Verification items for the finished model (mm, model axes). Face numbers are marked on the shaded views. A direction names the side the tool comes from. Coordinates: 2 decimals unless noted, no trailing zeros. Write each loop counter-clockwise with the first axis right and the second up, starting at its lowest first coordinate (ties: lowest second). Pieces come first, ordered by that corner, then holes. Notation, with made-up numbers: M 47.25,39.25 L 66.25,39.25 A24 ccw 66.25,66.25 Z; hole C 58.25,-12.75 d9. An arc over 180 degrees is marked long. Answer in a Markdown table with one row per item.
from build123d import *

# Parameters (mm, degrees)
EXTRUDE_1_DEPTH = 27.6


with BuildPart() as part:
    # 草图1 → 凸台-拉伸1 (new body)
    with BuildSketch(Plane.XY):
        with BuildLine():
            Line((13.366208682, 26.400087715), (20.217636418, 24.133453872))
            ThreePointArc((20.217636418, 24.133453872), (23.645978989, 21.408723367), (24.49520491, 17.112619964))
            Line((24.49520491, 17.112619964), (20.150640538, -10.351388685))
            ThreePointArc((20.150640538, -10.351388685), (17.326686466, -15.395594315), (11.903196789, -17.396715696))
            Line((11.903196789, -17.396715696), (-13.656803211, -17.396715696))
            ThreePointArc((-13.656803211, -17.396715696), (-19.080292887, -15.395594315), (-21.90424696, -10.351388685))
            Line((-21.90424696, -10.351388685), (-26.248811331, 17.112619964))
            ThreePointArc((-26.248811331, 17.112619964), (-25.422376853, 21.371021729), (-22.054699947, 24.105200178))
            Line((-22.054699947, 24.105200178), (-15.474583087, 26.383847403))
            ThreePointArc((-15.474583087, 26.383847403), (-14.885785491, 26.534208607), (-14.280201498, 26.584796429))
            Line((-14.280201498, 26.584796429), (12.219798502, 26.584796429))
            ThreePointArc((12.219798502, 26.584796429), (12.800395955, 26.538323396), (13.366208682, 26.400087715))
        make_face()
        with BuildLine():
            Line((12.533883483, 23.884191302), (19.385311219, 21.617557459))
            ThreePointArc((19.385311219, 21.617557459), (21.38292815, 20.029919212), (21.877752702, 17.526677859))
            Line((21.877752702, 17.526677859), (17.53318833, -9.93733079))
            ThreePointArc((17.53318833, -9.93733079), (15.605459203, -13.380680741), (11.903196789, -14.746715696))
            Line((11.903196789, -14.746715696), (-13.656803211, -14.746715696))
            ThreePointArc((-13.656803211, -14.746715696), (-17.359065624, -13.380680741), (-19.286794752, -9.93733079))
            Line((-19.286794752, -9.93733079), (-23.631359123, 17.526677859))
            ThreePointArc((-23.631359123, 17.526677859), (-23.149814624, 20.007951328), (-21.187546191, 21.601094677))
            Line((-21.187546191, 21.601094677), (-14.60742933, 23.879741901))
            ThreePointArc((-14.60742933, 23.879741901), (-14.446114921, 23.920936752), (-14.280201498, 23.934796429))
            Line((-14.280201498, 23.934796429), (12.219798502, 23.934796429))
            ThreePointArc((12.219798502, 23.934796429), (12.378866298, 23.922064091), (12.533883483, 23.884191302))
        make_face(mode=Mode.SUBTRACT)
    extrude(amount=EXTRUDE_1_DEPTH)


solid = part.part
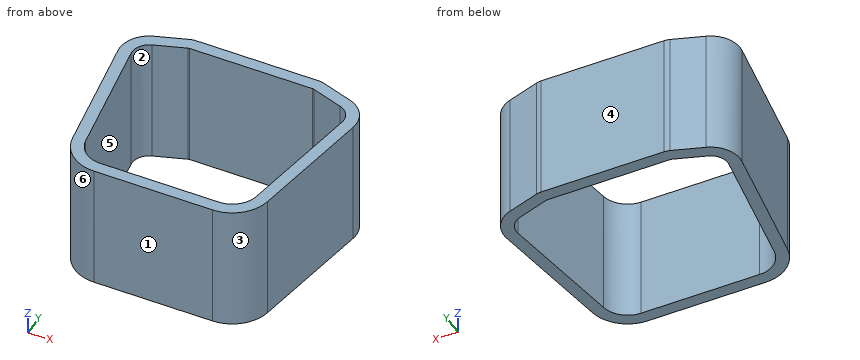
1) Sectioned sample at B-B (z = 3). Record the cut outline in (x, y).
Response values:
| item | result |
|---|---|
| outline | M -26.25,17.11 L -21.9,-10.35 A8.35 ccw -13.66,-17.4 L 11.9,-17.4 A8.35 ccw 20.15,-10.35 L 24.5,17.11 A6.35 ccw 20.22,24.13 L 13.37,26.4 A3.65 ccw 12.22,26.58 L -14.28,26.58 A3.65 ccw -15.47,26.38 L -22.05,24.11 A6.35 ccw Z; hole M -23.63,17.53 L -19.29,-9.94 A5.7 ccw -13.66,-14.75 L 11.9,-14.75 A5.7 ccw 17.53,-9.94 L 21.88,17.53 A3.7 ccw 19.39,21.62 L 12.53,23.88 A1 ccw 12.22,23.93 L -14.28,23.93 A1 ccw -14.61,23.88 L -21.19,21.6 A3.7 ccw Z |
2) Tool access check on the marked faces 1 and 2. Record the directions out of +Z, -Z, +X, -X, +Y, -Y that give a thin tool (end or side, any length) a straight path to the whole face; none if there is none.
Response values:
| item | result |
|---|---|
| face 1 | +Z, -Z, +X, -X, -Y |
| face 2 | +Z, -Z |
3) Release check for a two-part mould opening along X. For the marked faces 3, 4, 5 and 6 record: +X half, -X half, draft (parallel to the pull), parting line (faces both ways), or undercut.
Response values:
| item | result |
|---|---|
| face 3 | +X half |
| face 4 | draft |
| face 5 | undercut |
| face 6 | -X half |
4) Depth check by flat-ended pin: pin 1 (1.5 mm diameter, centred on y = 1, z = 12, fed in from -X); pin 2 (4 mm diameter, centred on y = -7.5, z = 19, fed in from -X); pin 3 (12 mm diameter, centred on y = -8, z = 4, fed in from +X). Enter the tip coordinate at first touch or a pass-through.
Response values:
| item | result |
|---|---|
| pin 1 | stops at x = -23.82 |
| pin 2 | stops at x = -22.67 |
| pin 3 | stops at x = 21.47 |
5) Sectioned sample at C-C (y = 20). Record the cut outline in (x, z).
Response values:
| item | result |
|---|---|
| outline | M -26.04,0 L -23.15,0 L -23.15,27.6 L -26.04,27.6 Z; M 21.4,0 L 24.28,0 L 24.28,27.6 L 21.4,27.6 Z |
6) Sectioned sample at A-A (x = 9). Record the cut outline in (y, z).
Response values:
| item | result |
|---|---|
| outline | M -17.4,0 L -14.75,0 L -14.75,27.6 L -17.4,27.6 Z; M 23.93,0 L 26.58,0 L 26.58,27.6 L 23.93,27.6 Z |
7) Thickness scan on L1, parallel to Y at x = 9.5, z = 12.75; L2, parallel to X at y = 14.5, z = 25; L3, parallel to Y at x = 15, z = 3. Record the ranges inside material, lowest first. Write a range as [from, to].
Response values:
| item | result |
|---|---|
| L1 | y = [-17.4, -14.75], [23.93, 26.58] |
| L2 | x = [-25.84, -23.15], [21.4, 24.08] |
| L3 | y = [-16.8, -13.83], [23.07, 25.86] |
